Could you check a few things on this model? Use its own coordinates, in mm. A direction names the side the tool comes from. Coordinates: 2 decimals unless noted, no trailing zeros. Write each loop counter-clockwise with the first axis right and the second up, starting at its lowest first coordinate (ties: lowest second). Pieces come first, ordered by that corner, then holes.
```python
from build123d import *

# Parameters (mm, degrees)
F2_DEPTH = 40
F3_DEPTH = 450
F3_TAPER = -2
F4_R     = 10


with BuildPart() as f2:
    # F0 (on Top) → F2 (new body)
    with BuildSketch(Plane.XY):
        with BuildLine():
            ThreePointArc((200, 170), (191.2132034356, 191.2132034356), (170, 200))
            Line((170, 200), (-170, 200))
            ThreePointArc((-170, 200), (-191.2132034356, 191.2132034356), (-200, 170))
            Line((-200, 170), (-200, -170))
            ThreePointArc((-200, -170), (-191.2132034356, -191.2132034356), (-170, -200))
            Line((-170, -200), (170, -200))
            ThreePointArc((170, -200), (191.2132034356, -191.2132034356), (200, -170))
            Line((200, -170), (200, 170))
        make_face()
    extrude(amount=F2_DEPTH)

    # F1 (on face) → F3 (join)
    with BuildSketch(Plane.XY):
        with BuildLine():
            Line((-175.1270698547, 120), (-147.8270698547, 120))
            ThreePointArc((-147.8270698547, 120), (-143.3369417942, 121.8598719395), (-141.4770698547, 126.35))
            Line((-141.4770698547, 126.35), (-141.4770698547, 153.65))
            ThreePointArc((-141.4770698547, 153.65), (-143.3369417942, 158.1401280605), (-147.8270698547, 160))
            Line((-147.8270698547, 160), (-175.1270698547, 160))
            ThreePointArc((-175.1270698547, 160), (-179.6171979153, 158.1401280605), (-181.4770698547, 153.65))
            Line((-181.4770698547, 153.65), (-181.4770698547, 126.35))
            ThreePointArc((-181.4770698547, 126.35), (-179.6171979153, 121.8598719395), (-175.1270698547, 120))
        make_face()
        with BuildLine():
            Line((-181.4770698547, -146.35), (-181.4770698547, -173.65))
            ThreePointArc((-181.4770698547, -173.65), (-179.6171979153, -178.1401280605), (-175.1270698547, -180))
            Line((-175.1270698547, -180), (-147.8270698547, -180))
            ThreePointArc((-147.8270698547, -180), (-143.3369417942, -178.1401280605), (-141.4770698547, -173.65))
            Line((-141.4770698547, -173.65), (-141.4770698547, -146.35))
            ThreePointArc((-141.4770698547, -146.35), (-143.3369417942, -141.8598719395), (-147.8270698547, -140))
            Line((-147.8270698547, -140), (-175.1270698547, -140))
            ThreePointArc((-175.1270698547, -140), (-179.6171979153, -141.8598719395), (-181.4770698547, -146.35))
        make_face()
        with BuildLine():
            Line((118.5229301453, 153.65), (118.5229301453, 126.35))
            ThreePointArc((118.5229301453, 126.35), (120.3828020847, 121.8598719395), (124.8729301453, 120))
            Line((124.8729301453, 120), (152.1729301453, 120))
            ThreePointArc((152.1729301453, 120), (156.6630582058, 121.8598719395), (158.5229301453, 126.35))
            Line((158.5229301453, 126.35), (158.5229301453, 153.65))
            ThreePointArc((158.5229301453, 153.65), (156.6630582058, 158.1401280605), (152.1729301453, 160))
            Line((152.1729301453, 160), (124.8729301453, 160))
            ThreePointArc((124.8729301453, 160), (120.3828020847, 158.1401280605), (118.5229301453, 153.65))
        make_face()
        with BuildLine():
            Line((118.5229301453, -146.35), (118.5229301453, -173.65))
            ThreePointArc((118.5229301453, -173.65), (120.3828020847, -178.1401280605), (124.8729301453, -180))
            Line((124.8729301453, -180), (152.1729301453, -180))
            ThreePointArc((152.1729301453, -180), (156.6630582058, -178.1401280605), (158.5229301453, -173.65))
            Line((158.5229301453, -173.65), (158.5229301453, -146.35))
            ThreePointArc((158.5229301453, -146.35), (156.6630582058, -141.8598719395), (152.1729301453, -140))
            Line((152.1729301453, -140), (124.8729301453, -140))
            ThreePointArc((124.8729301453, -140), (120.3828020847, -141.8598719395), (118.5229301453, -146.35))
        make_face()
    extrude(amount=F3_DEPTH, taper=F3_TAPER)

    # F4
    f4_edges = [f2.edges().sort_by_distance(p)[0] for p in [
        (200, 170, 20),
        (170, 200, 20),
        (191.213203, 191.213203, 0),
        (191.213203, 191.213203, 40),
    ]]
    fillet(f4_edges, radius=F4_R)


solid = f2.part
```
Item 1: If we mould it in two halves opening along Z, with no side actions, what happens to faces 5 (the flat face through (139, -161, 450)), 6 (the conical face through (-186, 116, 248)), 7 (the cylindrical face through (-191.445, -190.979, 19.86))? For each: released by +Z, released by -Z, zero draft, split by the parting line, or undercut.
Item 2: Will these pins go through, and if not, where does the flat tip stop? pin 1 Ø8 at (y, z) = (124, 122) entering from +X; pin 2 Ø8 at (y, z) = (104.5, 286) entering from +X; pin 3 Ø2 at (x, z) = (109, 390.5) entering from -Y; pin 4 Ø6 at (x, y) = (32, -101) entering from +Z.
Item 3: I want a section at B-B, the plane x = -2.5. List the corners of the cut face in (y, z) for me.
Item 4: If I drill on line 1 along Z through (x, y) = (-126.5, -72); line 2 along Y through (x, z) = (-149, 192.5); line 3 along Y through (x, z) = (136.5, 320), over which ranges is the centre line in solid material (lowest first)?
Item 5: I want a section at A-A, the plane z = 239.5. Count the separate pieces of the cut face and the enclosed holes in it, then the cut area to 3 significant figures.
Item 6: Which directions (+Z, -Z, +X, -X, +Y, -Y) give clear straight access to the entire face, cutting with the end or side of a thin tool? Please do faces 1 (the conical face through (-186, -184, 248)), 2 (the conical face through (162.9, 164.143, 247.87)), 3 (the conical face through (-137.1, -135.857, 247.87)), 4 (the conical face through (-137.334, -184.377, 247.87)).
Taken from the geometry:
1. face 5: released by +Z
1. face 6: undercut
1. face 7: zero draft
2. pin 1: stops at x = 162.9
2. pin 2: passes through
2. pin 3: stops at y = -187
2. pin 4: stops at z = 40
3. outline: (-200, 10) arc R10 ccw to (-190, 0) - (190, 0) arc R10 ccw to (200, 10) - (200, 30) arc R10 ccw to (190, 40) - (-190, 40) arc R10 ccw to (-200, 30) - close
4. line 1: z = 0 to 40
4. line 2: y = -186.72 to -133.28, 113.28 to 166.72
4. line 3: y = -191.17 to -128.83, 108.83 to 171.17
5. separate pieces: 4
5. enclosed holes: 0
5. area: 12,100 mm2
6. face 1: -X, -Y
6. face 2: +X, +Y
6. face 3: none
6. face 4: -Y
